Source: CAD feature listing. Evaluate the final solid. Frame: model axes, mm. Face numbers are marked on the shaded views. Round coordinates to 2 decimals unless told otherwise and drop trailing zeros. Order: outer loops, then holes, each group sorted by start corner. A loop starts at its lowest first (then second) coordinate and runs counter-clockwise, first axis right, second up.
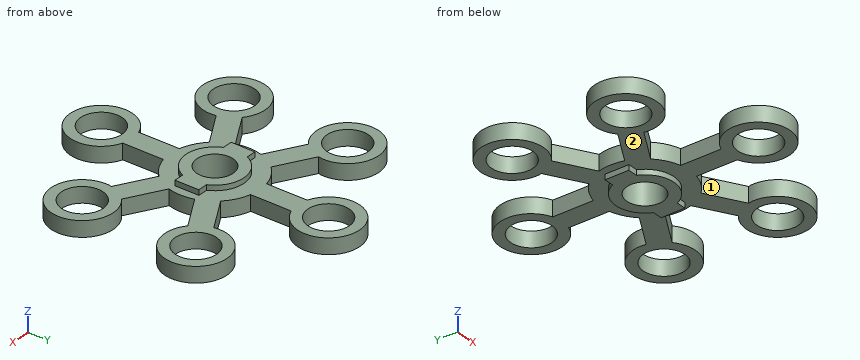
```python
from build123d import *

# Parameters (mm, degrees)
SKETCH2_R           = 17.5
BOSS_EXTRUDE2_DEPTH = 12.5
SKETCH2_5_R         = 20
BOSS_EXTRUDE5_DEPTH = 7.5


with BuildPart() as part:
    # Sketch2 → Boss-Extrude2 (new, symmetric)
    with BuildSketch(Plane.XY):
        with BuildLine():
            Line((25.529394822, 11.5), (35, 11.5))
            Line((35, 11.5), (35, -11.5))
            Line((35, -11.5), (25.529394822, -11.5))
            ThreePointArc((25.529394822, -11.5), (0, -28), (-25.529394822, -11.5))
            Line((-25.529394822, -11.5), (-35, -11.5))
            Line((-35, -11.5), (-35, 11.5))
            Line((-35, 11.5), (-25.529394822, 11.5))
            ThreePointArc((-25.529394822, 11.5), (0, 28), (25.529394822, 11.5))
        make_face()
        Circle(SKETCH2_R, mode=Mode.SUBTRACT)
    extrude(amount=BOSS_EXTRUDE2_DEPTH, both=True)

    # Sketch2<5> → Boss-Extrude5 (add, symmetric)
    with BuildSketch(Plane.XY):
        with BuildLine():
            Line((75.334884287, -31.947610338), (41.392953455, -12.351227436))
            ThreePointArc((41.392953455, -12.351227436), (43.196405116, 0), (41.392953455, 12.351227436))
            Line((41.392953455, 12.351227436), (75.334884287, 31.947610338))
            ThreePointArc((75.334884287, 31.947610338), (120.810543828, 69.75), (65.334884287, 49.268118414))
            Line((65.334884287, 49.268118414), (31.392953455, 29.671735512))
            ThreePointArc((31.392953455, 29.671735512), (21.598202558, 37.409184182), (10, 42.022962948))
            Line((10, 42.022962948), (10, 81.215728753))
            ThreePointArc((10, 81.215728753), (0, 139.5), (-10, 81.215728753))
            Line((-10, 81.215728753), (-10, 42.022962948))
            ThreePointArc((-10, 42.022962948), (-21.598202558, 37.409184182), (-31.392953455, 29.671735512))
            Line((-31.392953455, 29.671735512), (-65.334884287, 49.268118414))
            ThreePointArc((-65.334884287, 49.268118414), (-120.810543828, 69.75), (-75.334884287, 31.947610338))
            Line((-75.334884287, 31.947610338), (-41.392953455, 12.351227436))
            ThreePointArc((-41.392953455, 12.351227436), (-43.196405116, 0), (-41.392953455, -12.351227436))
            Line((-41.392953455, -12.351227436), (-75.334884287, -31.947610338))
            ThreePointArc((-75.334884287, -31.947610338), (-120.810543828, -69.75), (-65.334884287, -49.268118414))
            Line((-65.334884287, -49.268118414), (-31.392953455, -29.671735512))
            ThreePointArc((-31.392953455, -29.671735512), (-21.598202558, -37.409184182), (-10, -42.022962948))
            Line((-10, -42.022962948), (-10, -81.215728753))
            ThreePointArc((-10, -81.215728753), (0, -139.5), (10, -81.215728753))
            Line((10, -81.215728753), (10, -42.022962948))
            ThreePointArc((10, -42.022962948), (21.598202558, -37.409184182), (31.392953455, -29.671735512))
            Line((31.392953455, -29.671735512), (65.334884287, -49.268118414))
            ThreePointArc((65.334884287, -49.268118414), (120.810543828, -69.75), (75.334884287, -31.947610338))
        make_face()
        with Locations((0, 109.5)):
            Circle(SKETCH2_5_R, mode=Mode.SUBTRACT)
        with Locations((94.829781714, 54.75)):
            Circle(SKETCH2_5_R, mode=Mode.SUBTRACT)
        with Locations((94.829781714, -54.75)):
            Circle(SKETCH2_5_R, mode=Mode.SUBTRACT)
        with Locations((0, -109.5)):
            Circle(SKETCH2_5_R, mode=Mode.SUBTRACT)
        with Locations((-94.829781714, -54.75)):
            Circle(SKETCH2_5_R, mode=Mode.SUBTRACT)
        with Locations((-94.829781714, 54.75)):
            Circle(SKETCH2_5_R, mode=Mode.SUBTRACT)
        with BuildLine():
            ThreePointArc((25.529394822, 11.5), (0, 28), (-25.529394822, 11.5))
            Line((-25.529394822, 11.5), (-35, 11.5))
            Line((-35, 11.5), (-35, -11.5))
            Line((-35, -11.5), (-25.529394822, -11.5))
            ThreePointArc((-25.529394822, -11.5), (0, -28), (25.529394822, -11.5))
            Line((25.529394822, -11.5), (35, -11.5))
            Line((35, -11.5), (35, 11.5))
            Line((35, 11.5), (25.529394822, 11.5))
        make_face(mode=Mode.SUBTRACT)
    extrude(amount=BOSS_EXTRUDE5_DEPTH, both=True)


solid = part.part
```
1. Pull-direction query (X, two-part tool) for the marked faces 1 and 2; classes: released by +X, released by -X, zero draft, split by the parting line, or undercut.
2. First-contact query: pin 1 (12 mm diameter, centred on y = -45.5, z = -1.5, fed in from -X); pin 2 (7.5 mm diameter, centred on y = 65.5, z = 1.5, fed in from +X); pin 3 (12 mm diameter, centred on x = -10.5, y = 42.5, fed in from +Z). Flat tips, straight axial feed; report the tip coordinate or a pass-through.
3. Section B-B on x = 0. Return loops of the section in (y, z), plus the area to 3 significant figures.
4. Section C-C on z = -1.75. State how many separate pieces and enclosed holes the cut face has, plus the area to 3 significant figures.
5. Section A-A on y = 54.75. Return loops of the section in (x, z), plus the area to 3 significant figures.
6. Section D-D on y = -109.5. Return loops of the section in (x, z).
7. Line query: line 1 along Y through (x, z) = (0, -2.25); line 2 along X through (y, z) = (-56.5, -1.25); line 3 along Y through (x, z) = (-18, -2.5). Output: solid intervals per line, ascending.
Result:
1. face 1: undercut
1. face 2: zero draft
2. pin 1: stops at x = -124.65
2. pin 2: stops at x = 124
2. pin 3: stops at z = 7.5
3. outline: (-139.5, -7.5) - (-129.5, -7.5) - (-129.5, 7.5) - (-139.5, 7.5) - close; (-89.5, -7.5) - (-28, -7.5) - (-28, -12.5) - (-17.5, -12.5) - (-17.5, 12.5) - (-28, 12.5) - (-28, 7.5) - (-89.5, 7.5) - close; (17.5, -12.5) - (28, -12.5) - (28, -7.5) - (89.5, -7.5) - (89.5, 7.5) - (28, 7.5) - (28, 12.5) - (17.5, 12.5) - close; (129.5, -7.5) - (139.5, -7.5) - (139.5, 7.5) - (129.5, 7.5) - close
3. area: 2,670 mm2
4. separate pieces: 1
4. enclosed holes: 7
4. area: 18,800 mm2
5. outline: (-124.83, -7.5) - (-114.83, -7.5) - (-114.83, 7.5) - (-124.83, 7.5) - close; (-74.83, -7.5) - (-64.83, -7.5) - (-64.83, 7.5) - (-74.83, 7.5) - close; (-10, -7.5) - (10, -7.5) - (10, 7.5) - (-10, 7.5) - close; (64.83, -7.5) - (74.83, -7.5) - (74.83, 7.5) - (64.83, 7.5) - close; (114.83, -7.5) - (124.83, -7.5) - (124.83, 7.5) - (114.83, 7.5) - close
5. area: 900 mm2
6. outline: (-30, -7.5) - (-20, -7.5) - (-20, 7.5) - (-30, 7.5) - close; (20, -7.5) - (30, -7.5) - (30, 7.5) - (20, 7.5) - close
7. line 1: y = -139.5 to -129.5, -89.5 to -17.5, 17.5 to 89.5, 129.5 to 139.5
7. line 2: x = -124.78 to -114.75, -74.91 to -64.88, -10 to 10, 64.88 to 74.91, 114.75 to 124.78
7. line 3: y = -133.5 to -118.22, -100.78 to -85.5, -39.27 to 39.27, 85.5 to 100.78, 118.22 to 133.5
